Autodesk Inventor part; units mm, degrees
ref_plane "Arbeitsebene2" through (55.9, -6.9963, -17.125) normal (-1, 0, 0) x (0, 0, 1)
ref_plane "YZ Plane" through (0, 0, 0) normal (1, 0, 0) x (0, 1, 0)
ref_plane "XZ Plane" through (0, 0, 0) normal (0, 1, 0) x (-1, 0, 0)
ref_plane "Arbeitsebene1" through (0, 0, 0) normal (0, 0, 1) x (1, 0, 0)
sketch "Skizze1" plane through (0, 0, 0) normal (0, 0, 1) x (1, 0, 0)
  line L0 (8.6, 2.25) -> (8.6, -41.35)
  line L1 (8.6, -41.35) -> (-37.9, -41.35)
  line L2 (-37.9, -41.35) -> (-37.9, 2.25)
  line L3 (-37.9, 2.25) -> (8.6, 2.25)
  line L4 (9.6, 6.25) -> (-46.4, 6.25)
  line L5 (-46.4, 32.25) -> (-46.4, 6.25)
  line L6 (9.6, 32.25) -> (-46.4, 32.25)
  line L7 (9.6, 6.25) -> (9.6, 32.25)
  circle A0 centre (13.1, -11.2637) radius 1.4
  circle A1 centre (-42.4, -11.2637) radius 1.4
  circle A2 centre (-42.4, -31.25) radius 1.4
  line L8 (18.9, -41.35) -> (18.9, 19.75)
  line L9 (18.9, 19.75) -> (58.9, 19.75)
  line L10 (58.9, 19.75) -> (58.9, 19.25)
  line L11 (58.9, 19.25) -> (55.9, 19.25)
  line L12 (55.9, 17.6031) -> (55.9, 19.25)
  line L13 (63.9, 17.6031) -> (55.9, 17.6031)
  line L14 (63.9, 27.75) -> (63.9, 17.6031)
  arc A3 (63.9, 27.75) -> (58.9, 32.75) centre (58.9, 27.75) ccw
  line L15 (58.9, 32.75) -> (-58.9, 32.75)
  arc A4 (-58.9, 32.75) -> (-63.9, 27.75) centre (-58.9, 27.75) ccw
  line L16 (-63.9, -47.75) -> (-63.9, 27.75)
  arc A5 (-63.9, -47.75) -> (-58.9, -52.75) centre (-58.9, -47.75) ccw
  line L17 (-58.9, -52.75) -> (58.9, -52.75)
  arc A6 (58.9, -52.75) -> (63.9, -47.75) centre (58.9, -47.75) ccw
  line L18 (63.9, -47.75) -> (63.9, 0.8969)
  line L19 (55.9, 0.8969) -> (63.9, 0.8969)
  line L20 (55.9, -0.75) -> (55.9, 0.8969)
  line L21 (58.9, -0.75) -> (55.9, -0.75)
  line L22 (58.9, -0.75) -> (58.9, -1.25)
  line L23 (58.9, -1.25) -> (49.9, -1.25)
  line L24 (49.9, -1.25) -> (49.9, -41.35)
  line L25 (49.9, -41.35) -> (18.9, -41.35)
  circle A7 centre (13.1, 17.25) radius 1.4
  circle A8 centre (-50.2191, 17.25) radius 1.4
  line L26 (63.9, 17.6031) -> (63.9, 0.8969)
  line L27 (49.9, -1.25) -> (49.9, 19.75)
  line L28 (18.9, 6.25) -> (9.6, 6.25)
  line L29 (9.6, 6.25) -> (9.6, 2.25)
  line L30 (9.6, 2.25) -> (8.6, 2.25)
  line L31 (-37.9, 2.25) -> (-46.4, 2.25)
  line L32 (-46.4, 2.25) -> (-46.4, 6.25)
  line L33 (9.6, 32.25) -> (9.6, 32.75)
  line L34 (-46.4, 32.25) -> (-46.4, 32.75)
  circle A9 centre (58.9, 27.75) radius 1.4
  circle A10 centre (58.9, -47.75) radius 1.4
  circle A11 centre (-58.9, -47.75) radius 1.4
  circle A12 centre (-58.9, 27.75) radius 1.4
  line L35 (-46.4, 32.75) -> (9.6, 32.75)
  line L36 (9.6, 32.75) -> (9.6, 28.75)
  line L37 (9.6, 28.75) -> (-46.4, 28.75)
  line L38 (-46.4, 28.75) -> (-46.4, 32.75)
  point P0 (0, 0)
  point P1 (-46.4, 28.75)
  dimension "d0" = 2.8
  dimension "d1" = 2.8
  dimension "d2" = 2.8
  dimension "d3" = 2.8
  dimension "d29" = 4
extrude "Extrusion1" add sketch "Skizze1" along normal blind 5 contours L30 L29 L28 L8 L25 L24 L23 L22 L21 L20 L19 L18 A6 L17 A5 L16 A4 L15 L34 L5 L32 L31 L2 L1 L0 | L3 L31 L32 L4 L29 L30 | L7 L33 L15 A3 L14 L13 L12 L11 L10 L9 L8 L28 | L37 L5 L6 L7 | L6 L34 L15 L33 | L9 L10 L11 L12 L13 L26 L19 L20 L21 L22 L23 L27
sketch "Skizze2" plane through (0, 0, 5) normal (0, 0, 1) x (1, 0, 0)
  line L0 (-58.9, -52.75) -> (58.9, -52.75)
  line L1 (32.321, -52.75) -> (-27.679, -52.75)
  line L2 (-27.679, -52.75) -> (-27.679, -60.75)
  line L3 (-27.679, -60.75) -> (32.321, -60.75)
  line L4 (32.321, -60.75) -> (32.321, -52.75)
  circle A0 centre (27.321, -56.75) radius 2.25
  circle A1 centre (-22.679, -56.75) radius 2.25
  point P0 (0, 0)
  dimension "d6" = 60
  dimension "d7" = 8
  dimension "d8" = 4.5
  dimension "d9" = 4.5
  dimension "d10" = 5
  dimension "d11" = 50
extrude "Extrusion2" add sketch "Skizze2" against normal blind 3
fillet "Rundung1" radius 2 4 edges at (32.321, -60.75, 3.5) (32.321, -52.75, 3.5) (-27.679, -52.75, 3.5) (-27.679, -60.75, 3.5)
sketch "Skizze3" plane through (0, 0, 5) normal (0, 0, 1) x (1, 0, 0)
  arc A0 (-27.679, -58.75) -> (-25.679, -60.75) centre (-25.679, -58.75) ccw
  line L0 (-25.679, -60.75) -> (30.321, -60.75)
  arc A1 (30.321, -60.75) -> (32.321, -58.75) centre (30.321, -58.75) ccw
  line L1 (32.321, -58.75) -> (32.321, -54.75)
  arc A2 (34.321, -52.75) -> (32.321, -54.75) centre (34.321, -54.75) ccw
  line L2 (34.321, -52.75) -> (58.9, -52.75)
  arc A3 (58.9, -52.75) -> (63.9, -47.75) centre (58.9, -47.75) ccw
  line L3 (63.9, -47.75) -> (63.9, 27.75)
  arc A4 (63.9, 27.75) -> (58.9, 32.75) centre (58.9, 27.75) ccw
  line L4 (58.9, 32.75) -> (-58.9, 32.75)
  line L5 (9.6, 28.75) -> (9.6, 6.25)
  line L6 (9.6, 6.25) -> (-46.4, 6.25)
  line L7 (-46.4, 6.25) -> (-46.4, 28.75)
  arc A5 (-58.9, 32.75) -> (-63.9, 27.75) centre (-58.9, 27.75) ccw
  line L8 (-63.9, 27.75) -> (-63.9, -47.75)
  arc A6 (-63.9, -47.75) -> (-58.9, -52.75) centre (-58.9, -47.75) ccw
  line L9 (-58.9, -52.75) -> (-29.679, -52.75)
  arc A7 (-27.679, -54.75) -> (-29.679, -52.75) centre (-29.679, -54.75) ccw
  line L10 (-27.679, -54.75) -> (-27.679, -58.75)
  circle A8 centre (13.1, 17.25) radius 1.4
  circle A9 centre (58.9, 27.75) radius 1.4
  circle A10 centre (13.1, -11.2637) radius 1.4
  circle A11 centre (-42.4, -11.2637) radius 1.4
  circle A12 centre (-42.4, -31.25) radius 1.4
  circle A13 centre (-50.2191, 17.25) radius 1.4
  circle A14 centre (-58.9, 27.75) radius 1.4
  circle A15 centre (-58.9, -47.75) radius 1.4
  circle A16 centre (58.9, -47.75) radius 1.4
  line L11 (8.6, 2.25) -> (8.6, -41.35)
  line L12 (8.6, -41.35) -> (-37.9, -41.35)
  line L13 (-37.9, -41.35) -> (-37.9, 2.25)
  line L14 (-37.9, 2.25) -> (8.6, 2.25)
  line L15 (18.9, -41.35) -> (18.9, 19.75)
  line L16 (18.9, 19.75) -> (49.9, 19.75)
  line L17 (49.9, 19.75) -> (49.9, -41.35)
  line L18 (49.9, -41.35) -> (18.9, -41.35)
  circle A17 centre (-22.679, -56.75) radius 2.25
  circle A18 centre (27.321, -56.75) radius 2.25
  line L19 (-46.4, 28.75) -> (9.6, 28.75)
  point P0 (0, 0)
hole "Bohrung1" at (58.9, -47.75, 5) at (-58.9, -47.75, 5) at (-42.4, -31.25, 5) at (-42.4, -11.2637, 5) at (-50.2191, 17.25, 5) at (-58.9, 27.75, 5) at (13.1, -11.2637, 5) at (13.1, 17.25, 5) at (58.9, 27.75, 5) direction (0, 0, -1) diameter 2.9 end through all counterbore diameter 6.5 counterbore depth 3
ref_plane "Arbeitsebene2" through (55.9, -6.9963, -17.125) normal (-1, 0, 0) x (0, 0, 1)
sketch "Skizze4" plane through (49.9, -41.35, 0) normal (-1, 0, 0) x (0, 0, 1)
  line L0 (-10, 60) -> (0, 60)
  line L1 (-15.625, 40.6) -> (5, 40.6)
  line L2 (-17.125, 59.1) -> (-17.125, 42.1)
  line L3 (1.375, 40.6) -> (-15.625, 40.6)
  line L4 (-17.125, 42.1) -> (-17.125, 59.1)
  line L5 (-15.625, 60.6) -> (1.375, 60.6)
  line L6 (2.875, 59.1) -> (2.875, 42.1)
  line L7 (2.875, 40.6) -> (-17.125, 60.6) construction
  line L8 (-17.125, 40.6) -> (2.875, 60.6) construction
  arc A0 (-15.625, 60.6) -> (-17.125, 59.1) centre (-15.625, 59.1) ccw
  arc A1 (2.875, 59.1) -> (1.375, 60.6) centre (1.375, 59.1) ccw
  arc A2 (1.375, 40.6) -> (2.875, 42.1) centre (1.375, 42.1) ccw
  arc A3 (-17.125, 42.1) -> (-15.625, 40.6) centre (-15.625, 42.1) ccw
  arc A4 (-9, 49.9344) -> (-9, 51.2656) centre (-7.125, 50.6) ccw
  point P0 (0, 41.35)
  point P1 (-7.125, 50.6)
  point P2 (1.375, 40.6)
  dimension "d22" = 20
  dimension "d23" = 20
  dimension "d24" = 1.5
extrude "Extrusion3" cut sketch "Skizze4" against normal up to surface (6 mm away)
sketch "Skizze5" plane through (0, 0, 0) normal (0, 0, -1) x (-1, 0, 0)
  line L0 (-7.5796, -1.2774) -> (-17.8796, -1.2774)
  line L1 (38.1796, -41.35) -> (-32.748, -41.35)
  line L2 (-8.6, 2.25) -> (-8.6, -41.35)
  line L3 (-8.6, -41.35) -> (-18.6204, -41.35)
  line L4 (-7.5796, -1.2774) -> (-8.6, -1.2774)
  line L5 (-8.6, -1.2774) -> (-8.6, -41.35)
  line L6 (-18.6204, -41.35) -> (-21.2999, -41.35)
  line L7 (-21.2999, -41.35) -> (-21.2999, -21.25)
  line L8 (-21.2999, -21.25) -> (-18.6204, -21.25)
  line L9 (-49.6204, -13.9682) -> (-10.3204, -13.9682)
  line L10 (-8.6, 2.25) -> (-8.6, -41.35)
  line L11 (-8.6, -41.35) -> (-22.7391, -41.35)
  line L12 (-22.7391, -41.35) -> (-22.7391, -13.9682)
  line L13 (-22.7391, -13.9682) -> (-8.6, -13.9682)
  line L14 (-8.6, -13.9682) -> (-8.6, -41.35)
  point P0 (0, 0)
  point P1 (-8.6, -1.2774)
  point P2 (-8.6, -13.9682)
  point P3 (-22.7391, -13.9682)
extrude "Extrusion4" cut sketch "Skizze5" against normal blind 10
sketch "Skizze6" plane through (63.9, -47.75, 0) normal (1, 0, 0) x (0, 0, -1)
  arc A0 (3.0459, 50.3516) -> (3.0459, 63.6484) centre (7.125, 57) ccw
  circle A1 centre (7.125, 57) radius 8.5
  point P0 (0, 47.75)
  dimension "d30" = 17
extrude "Extrusion5" cut sketch "Skizze6" against normal blind 20
properties part number "11_Wellplatespacer"
Read the model definition and answer for the solid it produces. Units are mm, in the model's axes. A direction names the side the tool comes from. Coordinates: 2 decimals unless noted, no trailing zeros. Write each loop counter-clockwise with the first axis right and the second up, starting at its lowest first coordinate (ties: lowest second). Pieces come first, ordered by that corner, then holes. Notation, with made-up numbers: M 27.25,-20.75 L 45.25,-20.75 A14 cw 45.25,-4.75 Z; hole C 80.5,65 d11. An arc over 180 degrees is marked long. Use a Markdown table: item, result.
Q1. Straight lines are drawn through the part: L1, parallel to X at y = 19.5, z = 1.4; L2, parallel to X at y = -47.75, z = 1.1; L3, parallel to Y at x = -16, z = 2.8. For each, find the intervals that lie inside material, in ascending order. Write a range as [from, to].
Answer block:
| item | result |
|---|---|
| L1 | x = [-63.9, -46.4], [9.6, 18.9], [49.9, 63.9] |
| L2 | x = [-63.9, -60.35], [-57.45, 57.45], [60.35, 63.9] |
| L3 | y = [-60.75, -41.35], [2.25, 6.25], [28.75, 32.75] |
Q2. The part is cut by section D-D, the plane x = -42.4. Write down the section's boundary in (y, z), then the cut area to 3 significant figures.
Answer block:
| item | result |
|---|---|
| outline | M -52.75,0 L -32.7,0 L -32.7,2 L -34.5,2 L -34.5,5 L -52.75,5 Z; M -29.8,0 L -12.71,0 L -12.71,2 L -14.51,2 L -14.51,5 L -28,5 L -28,2 L -29.8,2 Z; M -9.81,0 L 6.25,0 L 6.25,5 L -8.01,5 L -8.01,2 L -9.81,2 Z; M 28.75,0 L 32.75,0 L 32.75,5 L 28.75,5 Z |
| area | 264 mm2 |
Q3. The part is cut by section A-A, the plane y = -56.75. Write down the section's boundary in (x, z), then the cut area to 3 significant figures.
Answer block:
| item | result |
|---|---|
| outline | M -27.68,2 L -24.93,2 L -24.93,5 L -27.68,5 Z; M -20.43,2 L 25.07,2 L 25.07,5 L -20.43,5 Z; M 29.57,2 L 32.32,2 L 32.32,5 L 29.57,5 Z |
| area | 153 mm2 |
Q4. Which of the six approach directions +Z, -Z, +X, -X, +Y, -Y give full straight-line access (tool end or side, diameter ignored) to faces 1 (the face through (13, -9, 0)), 2 (the face through (55.9, 9, 2)), 3 (the face through (13, 20.5, 3.5)), 4 (the face through (59.956, 9.319, 1.375)), 5 (the face through (18.9, 3, 2))?
Answer block:
| item | result |
|---|---|
| face 1 | -Z, +X, -X, +Y, -Y |
| face 2 | -Z |
| face 3 | +Z |
| face 4 | -Z, +X |
| face 5 | +Z, -Z |
Q5. Determine the mould class of faces 6 (the face through (-62.4, -51.32, 2.46)), 7 (the face through (-46.4, 18, 2)), 8 (the face through (2, -57, 2)) for opening direction Y: released by +Y, released by -Y, zero draft, split by the parting line, or undercut.
Answer block:
| item | result |
|---|---|
| face 6 | released by -Y |
| face 7 | undercut |
| face 8 | zero draft |
Q6. The part is cut by section B-B, the plane x = -3. Write down the section's boundary in (y, z).
Answer block:
| item | result |
|---|---|
| outline | M -60.75,2 L -52.75,2 L -52.75,0 L -41.35,0 L -41.35,5 L -60.75,5 Z; M 2.25,0 L 6.25,0 L 6.25,5 L 2.25,5 Z; M 28.75,0 L 32.75,0 L 32.75,5 L 28.75,5 Z |
Q7. The part is cut by section C-C, the plane y = -16. Write down the section's boundary in (x, z), then the cut area to 3 significant figures.
Answer block:
| item | result |
|---|---|
| outline | M -63.9,0 L -37.9,0 L -37.9,5 L -63.9,5 Z; M 49.9,0 L 63.9,0 L 63.9,5 L 49.9,5 Z |
| area | 200 mm2 |
Q8. Each of these flat-tipped pins is pushed along its axis until it touches: pin 1 Ø5 at (x, y) = (-43, -31) entering from +Z; pin 2 Ø5 at (x, y) = (27.321, -56.75) entering from -Z. Where does it stop, or does it pass through?
Answer block:
| item | result |
|---|---|
| pin 1 | stops at z = 2 |
| pin 2 | stops at z = 2 |
